The drawing under review shows one solid part. Ordinate dimensions are in mm from its lowest x, y, z. Give positions to 0.01 mm unless a question says otherwise; leave off trailing zeros. Write each loop counter-clockwise with the first axis right and the second up, starting at its lowest first coordinate (ties: lowest second). Pieces come first, ordered by that corner, then holes. Notation, with made-up numbers: (10, -7) - (65, -7) arc R20 ccw to (65, 26) - close; hole circle Ø8 at (78, 34). An arc over 180 degrees is marked (long way). Write item = value, one per line.
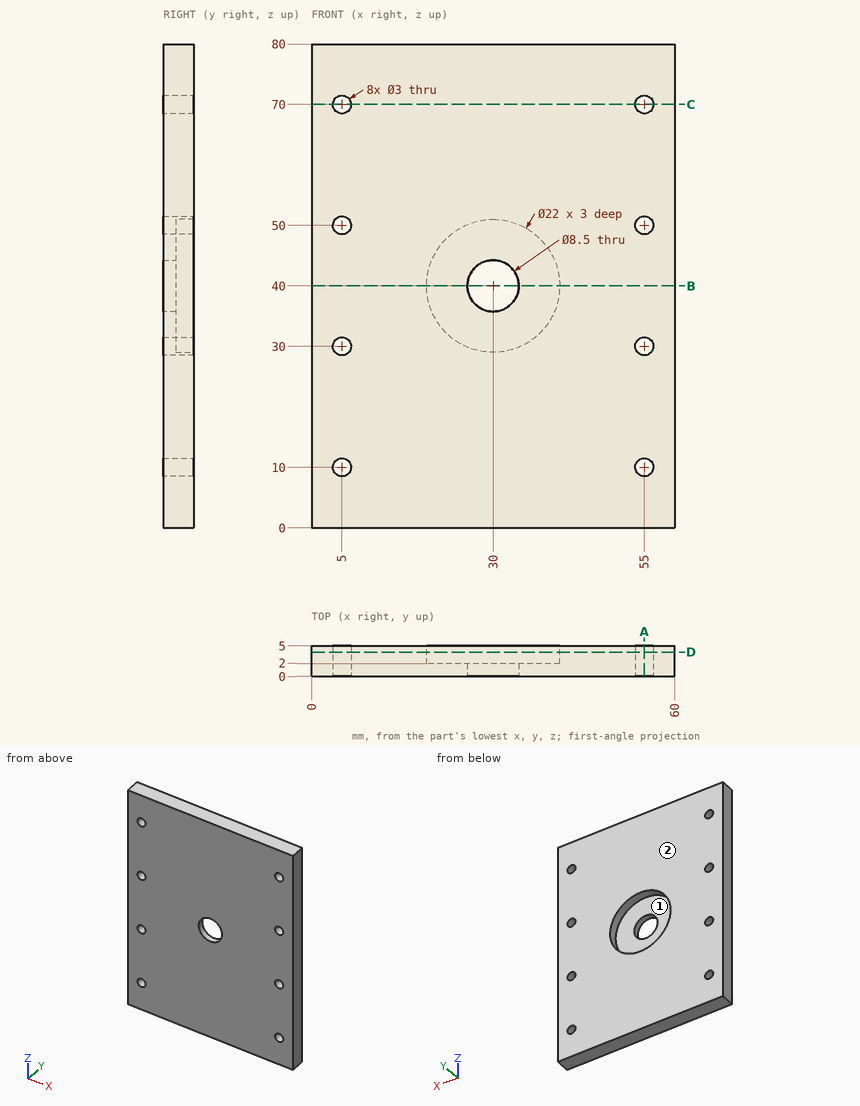
1. For line 1 (X direction, y = 2.45, z = 70); line 2 (X direction, y = 2.95, z = 30); line 3 (X direction, y = 3.3, z = 40), list the stretches that pass through material, from the lowest coordinate up. Write a range as from..to.
Findings below:
line_1 = 0..3.5, 6.5..53.5, 56.5..60
line_2 = 0..3.5, 6.5..25.42, 34.58..53.5, 56.5..60
line_3 = 0..19, 41..60
2. Draft analysis for pull direction X (two halves, no side actions). For the marked faces 1 and 2, state which applies: +X half, -X half, draft (parallel to the pull), parting line (faces both ways), or undercut.
Findings below:
face_1 = undercut
face_2 = draft
3. Insertion check: P1, Ø17.5, axis at x = 32, z = 39.5, coming from the +Y side. The pin has a flat end and moves straight along its axis. Give the tip position at first contact, or say it passes through.
Findings below:
P1 = 2
4. Take a section at D-D on y = 3.95. Count the separate pieces of the cut face and the enclosed holes in it, and give its area (3 significant figures).
Findings below:
separate_pieces = 1
enclosed_holes = 9
area = 4,360 mm²
5. Take a section at A-A on x = 55. Give the boundary of the cut face in (y, z).
Findings below:
outline = (0, 0) - (5, 0) - (5, 8.5) - (0, 8.5) - close; (0, 11.5) - (5, 11.5) - (5, 28.5) - (0, 28.5) - close; (0, 31.5) - (5, 31.5) - (5, 48.5) - (0, 48.5) - close; (0, 51.5) - (5, 51.5) - (5, 68.5) - (0, 68.5) - close; (0, 71.5) - (5, 71.5) - (5, 80) - (0, 80) - close
6. Take a section at C-C on z = 70. Give the boundary of the cut face in (x, y).
Findings below:
outline = (0, 0) - (3.5, 0) - (3.5, 5) - (0, 5) - close; (6.5, 0) - (53.5, 0) - (53.5, 5) - (6.5, 5) - close; (56.5, 0) - (60, 0) - (60, 5) - (56.5, 5) - close
7. Take a section at B-B on z = 40. Give the boundary of the cut face in (x, y).
Findings below:
outline = (0, 0) - (25.75, 0) - (25.75, 2) - (19, 2) - (19, 5) - (0, 5) - close; (34.25, 0) - (60, 0) - (60, 5) - (41, 5) - (41, 2) - (34.25, 2) - close
